from build123d import *

# Parameters (mm, degrees)
BOSS_EXTRUDE1_DEPTH   = 7
BOSS_EXTRUDE1_2_DEPTH = 7
BOSS_EXTRUDE2_DEPTH   = 2
SKETCH4_W             = 14
SKETCH4_H             = 9
BOSS_EXTRUDE3_DEPTH   = 0.5
SKETCH5_W             = 11
SKETCH5_H             = 7
CUT_EXTRUDE1_DEPTH    = 0.5
SKETCH6_W             = 24.5
SKETCH6_H             = 2
BOSS_EXTRUDE4_DEPTH   = 8
SKETCH7_W             = 24.5
SKETCH7_H             = 3
BOSS_EXTRUDE5_DEPTH   = 7
BOSS_EXTRUDE6_DEPTH   = 1


with BuildPart() as part:
    # Sketch1 → Boss-Extrude1 (new body)
    with BuildSketch(Plane(origin=(0, 0, 0), x_dir=(1, 0, 0), z_dir=(0, 1, 0))):
        Polygon((-38.972010623, -19.234572985), (-37.972010623, -19.234572985), (-37.972010623, -21.234572985), (-40.972010623, -21.234572985), (-40.972010623, -8.234572985), (-34.972010623, -8.234572985), (-34.972010623, -9.234572985), (-38.972010623, -9.234572985), align=None)
    extrude(amount=BOSS_EXTRUDE1_DEPTH)



with BuildPart() as body_2:
    # Sketch1 → Boss-Extrude1 2 (new body)
    with BuildSketch(Plane(origin=(0, 0, 0), x_dir=(1, 0, 0), z_dir=(0, 1, 0))):
        Polygon((-18.972010623, -19.234572985), (-18.972010623, -8.234572985), (-20.972010623, -8.234572985), (-20.972010623, -7.234572985), (-16.972010623, -7.234572985), (-16.972010623, -21.234572985), (-19.972010623, -21.234572985), (-19.972010623, -19.234572985), align=None)
    extrude(amount=BOSS_EXTRUDE1_2_DEPTH)


with BuildPart() as part_1:
    add(part.part)

    add(body_2.part)  # Boss-Extrude2 merges body 2
    # Sketch2 → Boss-Extrude2 (add)
    with BuildSketch(Plane.XZ):
        Polygon((-40.972010623, 21.234572985), (-16.972010623, 21.234572985), (-16.972010623, 7.234572985), (-28.972010623, 7.234572985), (-30.273567276, 8.234572985), (-40.972010623, 8.234572985), align=None)
    extrude(amount=BOSS_EXTRUDE2_DEPTH)

    # Sketch4 → Boss-Extrude3 (add)
    with BuildSketch(Plane(origin=(-16.972010623, 0, 0), x_dir=(0, 0, -1), z_dir=(1, 0, 0))):
        with Locations((-14.234572985, 2.5)):
            Rectangle(SKETCH4_W, SKETCH4_H)
    extrude(amount=BOSS_EXTRUDE3_DEPTH)

    # Sketch5 → Cut-Extrude1 (cut)
    with BuildSketch(Plane.ZY.offset(18.972010623)):
        with Locations((13.734572985, 3.5)):
            Rectangle(SKETCH5_W, SKETCH5_H)
    extrude(amount=-CUT_EXTRUDE1_DEPTH, mode=Mode.SUBTRACT)

    # Sketch6 → Boss-Extrude4 (add)
    with BuildSketch(Plane.XY.offset(21.234572985)):
        with Locations((-28.722010623, -1)):
            Rectangle(SKETCH6_W, SKETCH6_H)
    extrude(amount=BOSS_EXTRUDE4_DEPTH)

    # Sketch7 → Boss-Extrude5 (add)
    with BuildSketch(Plane(origin=(0, 0, 0), x_dir=(1, 0, 0), z_dir=(0, 1, 0))):
        with Locations((-28.722010623, -27.734572985)):
            Rectangle(SKETCH7_W, SKETCH7_H)
    extrude(amount=BOSS_EXTRUDE5_DEPTH)

    # Sketch8 → Boss-Extrude6 (add)
    with BuildSketch(Plane.XZ.offset(2)):
        Polygon((-40.972010623, 29.234572985), (-40.972010623, 8.234572985), (-30.273567276, 8.234572985), (-28.972010623, 7.234572985), (-16.472010623, 7.234572985), (-16.472010623, 29.234572985), align=None)
    extrude(amount=BOSS_EXTRUDE6_DEPTH)


solid = part_1.part
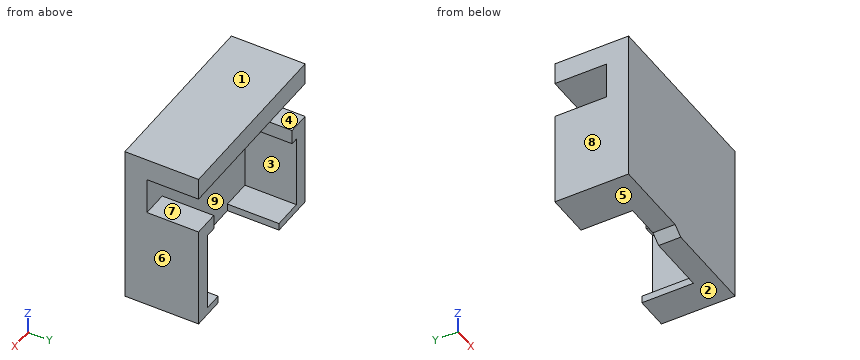
Can you work these out from the model? Positions are in its coordinate system, mm. Face numbers are marked on the shaded views. A direction names the side the tool comes from. Round coordinates to 2 decimals unless told otherwise and drop trailing zeros. Loops run counter-clockwise (first coordinate to the right, second up) from the corner with the lowest first, then second, coordinate; pieces in that order, holes last. Notation, with made-up numbers: (37, -32) - (91, -32) arc R15 ccw to (91, -6) - close; hole circle Ø6 at (71, -29.75). An arc over 180 degrees is marked (long way). Answer in a Markdown table with one row per item. Add a question column.
Q1. I want a section at C-C on z = 16. List the corners of the cut face in (x, y) for me, and give its area (4 significant figures).
Q2. We'd pull the mould along X, two halves only. Please class the marked faces 6, 7, 8 and 9: pulls with the +X half, pulls with the -X half, needs draft (parallel to the pull), parting line crosses it, or undercut.
Q3. I want a section at D-D on y = -1.5. List the corners of the cut face in (x, z) for me, and give its area (3 significant figures).
Q4. I want a section at B-B on x = -37.5. List the corners of the cut face in (y, z) for me.
Q5. I need wall thicknesses on L1, parallel to X at y = 3, z = 14.25; L2, parallel to X at y = 4.5, z = 21; L3, parallel to Z at x = -36.75, y = 2.75. Which ranges of each line are inside material? Lowest first, please.
Q6. Which directions (+Z, -Z, +X, -X, +Y, -Y) give clear straight access to the entire face, cutting with the end or side of a thin tool? Please do the marked faces 1, 2, 3, 4 and 5.
Q7. I want a section at A-A on y = 4.5. List the corners of the cut face in (x, z) for me.
Q8. For pin 1 Ø3 at (x, y) = (-31, 5) entering from -Z; pin 2 Ø1.1 at (x, y) = (-38.5, 2) entering from -Z; pin 3 Ø0.5 at (y, z) = (4, 7.5) entering from -X, each with a flat end and sliding along its axis, tell me the tip position at first contact or that it passes through.
A:
| question | item | result |
|---|---|---|
| 1 | outline | (-40.97, -3) - (-16.47, -3) - (-16.47, 7) - (-18.47, 7) - (-18.47, 0) - (-38.97, 0) - (-38.97, 7) - (-40.97, 7) - close |
| 1 | area | 101.5 mm^2 |
| 2 | face 6 | pulls with the +X half |
| 2 | face 7 | needs draft |
| 2 | face 8 | pulls with the -X half |
| 2 | face 9 | undercut |
| 3 | outline | (-40.97, 8.23) - (-30.27, 8.23) - (-28.97, 7.23) - (-16.47, 7.23) - (-16.47, 29.23) - (-40.97, 29.23) - close |
| 3 | area | 528 mm^2 |
| 4 | outline | (-3, 8.23) - (7, 8.23) - (7, 9.23) - (0, 9.23) - (0, 26.23) - (7, 26.23) - (7, 29.23) - (-3, 29.23) - close |
| 5 | L1 | -40.97 to -38.97, -18.47 to -16.47 |
| 5 | L2 | -40.97 to -37.97, -19.97 to -16.47 |
| 5 | L3 | 8.23 to 9.23, 26.23 to 29.23 |
| 6 | face 1 | +Z, +X, -X, +Y, -Y |
| 6 | face 2 | -Z, +X, -X, +Y, -Y |
| 6 | face 3 | +Y |
| 6 | face 4 | +X, -X, +Y |
| 6 | face 5 | -Z, -X, +Y, -Y |
| 7 | outline | (-40.97, 8.23) - (-34.97, 8.23) - (-34.97, 9.23) - (-38.97, 9.23) - (-38.97, 19.23) - (-37.97, 19.23) - (-37.97, 21.23) - (-40.97, 21.23) - close; (-40.97, 26.23) - (-16.47, 26.23) - (-16.47, 29.23) - (-40.97, 29.23) - close; (-20.97, 7.23) - (-16.47, 7.23) - (-16.47, 21.23) - (-19.97, 21.23) - (-19.97, 19.23) - (-18.47, 19.23) - (-18.47, 8.23) - (-20.97, 8.23) - close |
| 8 | pin 1 | z = 26.23 |
| 8 | pin 2 | z = 8.23 |
| 8 | pin 3 | x = -20.97 |
